```python
from build123d import *

# Parameters (mm, degrees)
SKETCH1_R                 = 6.35
BOSS_EXTRUDE1_DEPTH       = 101.6
M5X0_8_TAPPED_HOLE1_D     = 4.2
M5X0_8_TAPPED_HOLE1_DEPTH = 25.4
M5X0_8_TAPPED_HOLE1_TIP   = 1.2618073
FILLET1_R                 = 1.27


with BuildPart() as part:
    # Sketch1 → Boss-Extrude1 (new body)
    with BuildSketch(Plane.XY):
        Circle(SKETCH1_R)
    extrude(amount=BOSS_EXTRUDE1_DEPTH)

    # M5x0.8 Tapped Hole1
    with Locations(Plane(origin=(0, 0, 0), x_dir=(-1, 0, 0), z_dir=(0, 0, -1))):
        with Locations((0, 0)):
            Hole(M5X0_8_TAPPED_HOLE1_D / 2, depth=M5X0_8_TAPPED_HOLE1_DEPTH)
            with Locations((0, 0, -(M5X0_8_TAPPED_HOLE1_DEPTH + M5X0_8_TAPPED_HOLE1_TIP / 2))):  # 118° drill point
                Cone(0, M5X0_8_TAPPED_HOLE1_D / 2, M5X0_8_TAPPED_HOLE1_TIP, mode=Mode.SUBTRACT)

    # Fillet1
    fillet1_edges = [part.edges().sort_by_distance(p)[0] for p in [
        (-6.35, 0, 101.6),
    ]]
    fillet(fillet1_edges, radius=FILLET1_R)


solid = part.part
```
Verification items for the finished model (mm, model axes). A direction names the side the tool comes from. Coordinates: 2 decimals unless noted, no trailing zeros. Loops run counter-clockwise (first coordinate to the right, second up) from the corner with the lowest first, then second, coordinate; pieces in that order, holes last. Notation, with made-up numbers: (-26, 41) -> (17, 41) arc R21 cw to (17, 70) -> close; hole circle Ø7 at (-29, 16.25). An arc over 180 degrees is marked (long way). Put each result on its own line as item: value.
1. Thickness scan on line 1 (Y direction, x = 0, z = 17); line 2 (X direction, y = -0.5, z = 59.5); line 3 (Y direction, x = 2.75, z = 7.5). Record the ranges inside material, lowest first.
Result set:
line 1: y = -6.35 to -2.1, 2.1 to 6.35
line 2: x = -6.33 to 6.33
line 3: y = -5.72 to 5.72
2. Tool access check on faces 4 (the face through (-2, 2, 0)), 5 (the face through (2.003, 0.631, 12.878)). Record the directions out of +Z, -Z, +X, -X, +Y, -Y that give a thin tool (end or side, any length) a straight path to the whole face; none if there is none.
Result set:
face 4: -Z, +X, -X, +Y, -Y
face 5: -Z
3. Gauge pin test, flat ends, axial feed: P1, Ø3, axis at x = -2.5, z = 81.5, coming from the +Y side; P2, Ø5, axis at x = -4.5, z = 12.5, coming from the -Y side; P3, Ø4, axis at y = -3, z = 33, coming from the +X side. Record the tip position at first contact, or that the pin passes through.
Result set:
P1: stops at y = 6.27
P2: stops at y = -6.03
P3: stops at x = 6.27
4. Mould release check, pull along Y, two halves, no side actions. Record for faces 1 (the face through (-0.35, 0.11, 26.44)), 2 (the face through (-1.38, -6.2, 49.46)), 3 (the face through (0, 0, 101.6)): pulls with the +Y half, pulls with the -Y half, needs draft (parallel to the pull), parting line crosses it, or undercut.
Result set:
face 1: undercut
face 2: parting line crosses it
face 3: needs draft
5. Section check A-A, the plane z = 39.5. Record the boundary of the cut face in (x, y).
Result set:
outline: circle Ø12.7 at (0, 0)
